Autodesk Inventor part; units mm, degrees
ref_plane "YZ Plane" through (0, 0, 0) normal (1, 0, 0) x (0, 1, 0)
ref_plane "XZ Plane" through (0, 0, 0) normal (0, 1, 0) x (-1, 0, 0)
ref_plane "XY Plane" through (0, 0, 0) normal (0, 0, 1) x (1, 0, 0)
sketch "Skizze1" plane through (0, 0, 0) normal (0, 1, 0) x (-1, 0, 0)
  line L0 (0, 0) -> (-25.5, 0)
  line L1 (-25.5, 0) -> (-25.5, 9)
  line L2 (-25.5, 9) -> (0, 9)
  line L3 (0, 9) -> (0, 0)
  dimension "d0" = 25.5
  dimension "d1" = 9
extrude "Extrusion1" add sketch "Skizze1" along normal blind 5.5
sketch "Skizze2" plane through (0, 0, 0) normal (0, -1, 0) x (1, 0, 0)
  line L0 (25.5, 0) -> (0, 0)
  arc A0 (19.75, 0) -> (5.75, 0) centre (12.75, 0) ccw
  dimension "d4" = 14
extrude "Extrusion2" cut sketch "Skizze2" against normal through all
sketch "Skizze5" plane through (0, 0, 9) normal (0, 0, 1) x (1, 0, 0)
  line L0 (0, 0) -> (0, 5.5) construction
  line L1 (0, 2.75) -> (25.5934, 2.75) construction
  line L2 (25.5, 0) -> (0, 0) construction
  line L3 (12.75, 0) -> (12.75, 5.5) construction
  line L4 (0, 5.5) -> (25.5, 5.5) construction
  point P0 (2.8, 2.75)
  point P1 (22.7, 2.75)
  dimension "d33" = 2.8
hole "Bohrung4" at (2.8, 2.75, 9) at (22.7, 2.75, 9) direction (0, 0, -1) diameter 3.3 end through all
fillet "Rundung1" radius 2 4 edges at (25.5, 0, 4.5) (25.5, 5.5, 4.5) (0, 0, 4.5) (0, 5.5, 4.5)
properties part number "Wellenhalterung_oben" material "ABS-Kunststoff"
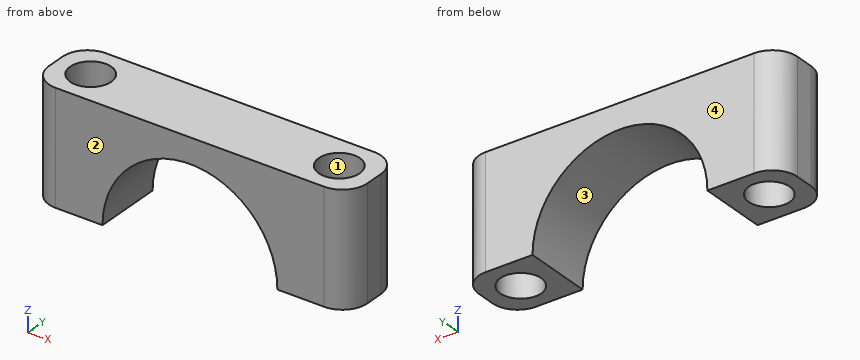
For this review, take the finished solid that the model builds, in its own axes (mm). Face numbers are marked on the shaded views. Coordinates: 2 decimals unless noted, no trailing zeros. Order: outer loops, then holes, each group sorted by start corner. A loop starts at its lowest first (then second) coordinate and runs counter-clockwise, first axis right, second up. Notation, with made-up numbers: (41.5, 84.5) -> (52.5, 84.5) arc R23 ccw to (52.5, 111.5) -> close; hole circle Ø1 at (-37.5, -6). An arc over 180 degrees is marked (long way). Use CSV: the item, a comma, the result in double quotes. Start each with the question number.
Item 1: We need section D-D, the plane z = 2.25. Give the boundary of the cut face in (x, y), then the cut area to 3 significant figures.
Item 2: We need section B-B, the plane z = 5.25. Give the boundary of the cut face in (x, y), then the cut area to 3 significant figures.
Item 3: We need section C-C, the plane x = 2.8. Give the boundary of the cut face in (y, z), then the cut area to 3 significant figures.
Item 4: Wall thickness on probe 1 along Y at (x, z) = (2.8, 2.5); probe 2 along X at (y, z) = (3.25, 5.75); probe 3 along X at (y, z) = (2.75, 3.5): over which ranges is each line inside the solid? List them lowest first.
Item 5: Draft analysis for pull direction Y (two halves, no side actions). For the marked faces 1, 2, 3 and 4, state which applies: pulls with the +Y half, pulls with the -Y half, needs draft (parallel to the pull), parting line crosses it, or undercut.
Item 6: We need section A-A, the plane y = 2.75. Give the boundary of the cut face in (x, z), then the cut area to 3 significant figures.
Derived:
1,outline,"(0, 2) arc R2 ccw to (2, 0) -> (6.12, 0) -> (6.12, 5.5) -> (2, 5.5) arc R2 ccw to (0, 3.5) -> close; (19.38, 0) -> (23.5, 0) arc R2 ccw to (25.5, 2) -> (25.5, 3.5) arc R2 ccw to (23.5, 5.5) -> (19.38, 5.5) -> close; hole circle Ø3.3 at (2.8, 2.75); hole circle Ø3.3 at (22.7, 2.75)"
1,area,"46.8 mm^2"
2,outline,"(0, 2) arc R2 ccw to (2, 0) -> (8.12, 0) -> (8.12, 5.5) -> (2, 5.5) arc R2 ccw to (0, 3.5) -> close; (17.38, 0) -> (23.5, 0) arc R2 ccw to (25.5, 2) -> (25.5, 3.5) arc R2 ccw to (23.5, 5.5) -> (17.38, 5.5) -> close; hole circle Ø3.3 at (2.8, 2.75); hole circle Ø3.3 at (22.7, 2.75)"
2,area,"68.8 mm^2"
3,outline,"(0, 0) -> (1.1, 0) -> (1.1, 9) -> (0, 9) -> close; (4.4, 0) -> (5.5, 0) -> (5.5, 9) -> (4.4, 9) -> close"
3,area,"19.8 mm^2"
4,probe 1,"y = 0 to 1.1, 4.4 to 5.5"
4,probe 2,"x = 0 to 1.23, 4.37 to 8.76, 16.74 to 21.13, 24.27 to 25.5"
4,probe 3,"x = 0 to 1.15, 4.45 to 6.69, 18.81 to 21.05, 24.35 to 25.5"
5,face 1,"undercut"
5,face 2,"pulls with the -Y half"
5,face 3,"needs draft"
5,face 4,"pulls with the +Y half"
6,outline,"(0, 0) -> (1.15, 0) -> (1.15, 9) -> (0, 9) -> close; (4.45, 0) -> (5.75, 0) arc R7 cw to (19.75, 0) -> (21.05, 0) -> (21.05, 9) -> (4.45, 9) -> close; (24.35, 0) -> (25.5, 0) -> (25.5, 9) -> (24.35, 9) -> close"
6,area,"93.1 mm^2"
